```python
from build123d import *

# Parameters (mm, degrees)
SKETCH1_W                 = 130
SKETCH1_H                 = 110
BOSS_EXTRUDE1_DEPTH       = 145
SHELL2_T                  = -5
SHELL2_THICKNESS_2_FACE_W = 100
SHELL2_THICKNESS_2_FACE_H = 120
SHELL2_THICKNESS_2_DEPTH  = 5
SKETCH2_R                 = 23
BOSS_EXTRUDE2_DEPTH       = 12
SKETCH2_3_R               = 25
BOSS_EXTRUDE3_DEPTH       = 13
SKETCH3_R                 = 16
CUT_EXTRUDE1_DEPTH        = 10
SKETCH4_R                 = 17.5
CUT_EXTRUDE4_DEPTH        = 11
SKETCH5_R                 = 5.5
SKETCH5_R_2               = 7
CUT_EXTRUDE5_DEPTH        = 194.261480901
SKETCH7_R                 = 4.25
CUT_EXTRUDE6_DEPTH        = 10
FILLET1_R                 = 3
FILLET2_R                 = 2


with BuildPart() as part:
    # Sketch1 → Boss-Extrude1 (new body)
    with BuildSketch(Plane(origin=(0, 0, 0), x_dir=(0, 1, 0), z_dir=(0, 0, 1))):
        Rectangle(SKETCH1_W, SKETCH1_H)
    extrude(amount=BOSS_EXTRUDE1_DEPTH)

    # Shell2
    shell2_openings = [part.faces().sort_by_distance(p)[0] for p in [
        (0, 0, 145),
    ]]
    offset(amount=SHELL2_T, openings=shell2_openings, kind=Kind.INTERSECTION)

    # Shell2 thickness 2 face (on inner face of the shell) → Shell2 thickness 2 (add)
    with BuildSketch(Plane(origin=(0, 0, 5), x_dir=(-1, 0, 0), z_dir=(0, 0, -1))):
        Rectangle(SHELL2_THICKNESS_2_FACE_W, SHELL2_THICKNESS_2_FACE_H)
    extrude(amount=-SHELL2_THICKNESS_2_DEPTH)

    # Sketch2 → Boss-Extrude2 (add)
    with BuildSketch(Plane.YZ.offset(-50)):
        with Locations((-31, 75)):
            Circle(SKETCH2_R)
    boss_extrude2 = extrude(amount=BOSS_EXTRUDE2_DEPTH)

    # Sketch2_3 → Boss-Extrude3 (add)
    with BuildSketch(Plane.YZ.offset(-50)):
        with Locations(Location((23, 75, 0), (0, 0, 180))):
            Circle(SKETCH2_3_R)
    boss_extrude3 = extrude(amount=BOSS_EXTRUDE3_DEPTH)

    # Sketch3 → Cut-Extrude1 (cut)
    with BuildSketch(Plane.YZ.offset(-38)):
        with Locations((-31, 75)):
            Circle(SKETCH3_R)
    cut_extrude1 = extrude(amount=-CUT_EXTRUDE1_DEPTH, mode=Mode.SUBTRACT)

    # Sketch4 → Cut-Extrude4 (cut)
    with BuildSketch(Plane.YZ.offset(-37)):
        with Locations((23, 75)):
            Circle(SKETCH4_R)
    cut_extrude4 = extrude(amount=-CUT_EXTRUDE4_DEPTH, mode=Mode.SUBTRACT)

    # Mirror1: Boss-Extrude2, Boss-Extrude3, Cut-Extrude1, Cut-Extrude4 across plane
    add(boss_extrude2.mirror(Plane(origin=(0, 0, 0), x_dir=(0, 0, 1), z_dir=(1, 0, 0))))
    add(boss_extrude3.mirror(Plane(origin=(0, 0, 0), x_dir=(0, 0, 1), z_dir=(1, 0, 0))))
    add(cut_extrude1.mirror(Plane(origin=(0, 0, 0), x_dir=(0, 0, 1), z_dir=(1, 0, 0))), mode=Mode.SUBTRACT)
    add(cut_extrude4.mirror(Plane(origin=(0, 0, 0), x_dir=(0, 0, 1), z_dir=(1, 0, 0))), mode=Mode.SUBTRACT)

    # Sketch5 → Cut-Extrude5 (cut, through all)
    with BuildSketch(Plane(origin=(-55, 0, 0), x_dir=(0, -1, 0), z_dir=(-1, 0, 0))):
        with Locations((31, 75)):
            Circle(SKETCH5_R)
        with Locations((-23, 75)):
            Circle(SKETCH5_R_2)
    extrude(amount=-CUT_EXTRUDE5_DEPTH, mode=Mode.SUBTRACT)

    # Sketch7 → Cut-Extrude6 (cut)
    with BuildSketch(Plane(origin=(0, 0, 0), x_dir=(1, 0, 0), z_dir=(0, 0, -1))):
        with Locations(Location((-40, 50, 0), (0, 0, 180))):
            Circle(SKETCH7_R)
        with Locations(Location((40, 50, 0), (0, 0, 180))):
            Circle(SKETCH7_R)
        with Locations(Location((-40, -50, 0), (0, 0, 180))):
            Circle(SKETCH7_R)
        with Locations(Location((40, -50, 0), (0, 0, 180))):
            Circle(SKETCH7_R)
    extrude(amount=-CUT_EXTRUDE6_DEPTH, mode=Mode.SUBTRACT)

    # Fillet1
    fillet1_edges = [part.edges().sort_by_distance(p)[0] for p in [
        (-50, -60, 77.5),
        (50, -60, 77.5),
        (50, 60, 77.5),
        (-50, 60, 77.5),
        (-55, -65, 72.5),
        (-55, 65, 72.5),
        (55, 65, 72.5),
        (55, -65, 72.5),
    ]]
    fillet(fillet1_edges, radius=FILLET1_R)

    # Fillet2
    fillet2_edges = [part.edges().sort_by_distance(p)[0] for p in [
        (-38, -54, 75),
        (-37, 48, 75),
        (38, -54, 75),
        (37, 48, 75),
    ]]
    fillet(fillet2_edges, radius=FILLET2_R)


solid = part.part
```
Design review of the part built by this model. Coordinates are the model's own, in mm. A direction names the side the tool comes from. Coordinates: 2 decimals unless noted, no trailing zeros. Order: outer loops, then holes, each group sorted by start corner. A loop starts at its lowest first (then second) coordinate and runs counter-clockwise, first axis right, second up. Notation, with made-up numbers: (30, 24) -> (40, 24) arc R27 ccw to (40, 44) -> close; hole circle Ø9 at (39.5, -18.5). An arc over 180 degrees is marked (long way). One line per item, written item: value. Start each with the question number.
Q1. Take a section at B-B, the plane y = 50. State the section outline as (x, z) points.
Q2. Insertion check: pin 1 Ø12.5 at (y, z) = (23, 75) entering from -X; pin 2 Ø6 at (x, y) = (-3.5, -24.5) entering from +Z. Each pin has a flat end and moves straight along its axis. Give the tip position at first contact, or say it passes through.
Q3. Take a section at D-D, the plane x = -26. State the section outline as (y, z) points.
Q4. Take a section at C-C, the plane z = 34.5. State the section outline as (x, y) points, then the cut area to 3 significant figures.
Q5. Take a section at A-A, the plane x = 42. State the section outline as (y, z) points.
Q6. Mouldability with a two-part tool opening along Y and no side actions: class faces 1 (the flat face through (1, 65, 71)), 2 (the cylindrical face through (42.93, -33.083, 90.864)), 3 (the flat face through (48, 31, 75)), 4 (the flat face through (55, -1, 71)) as pulls with the +Y half, pulls with the -Y half, needs draft (parallel to the pull), parting line crosses it, or undercut.
Q7. Tool access review of faces 5 (the cylindrical face through (-44.577, 47.976, 73.901)), 6 (the flat face through (37, 31.63, 59.56)), 7 (the cylindrical face through (-36.63, 47.41, 4.93)): name each direction out of +Z, -Z, +X, -X, +Y, -Y from which nothing blocks a thin tool from reaching the whole face with its end or side.
Q8. For probe 1 along Y at (x, z) = (-40, 3); probe 2 along Z at (x, y) = (-44, -31); probe 3 along Y at (x, z) = (-19, 90), list the stretches that pass through material, from the lowest coordinate up.
Values follow:
1. outline: (-55, 0) -> (-44.25, 0) -> (-44.25, 10) -> (-50, 10) -> (-50, 145) -> (-55, 145) -> close; (-35.75, 0) -> (35.75, 0) -> (35.75, 10) -> (-35.75, 10) -> close; (44.25, 0) -> (55, 0) -> (55, 145) -> (50, 145) -> (50, 10) -> (44.25, 10) -> close
2. pin 1: passes through
2. pin 2: stops at z = 10
3. outline: (-65, 0) -> (65, 0) -> (65, 145) -> (60, 145) -> (60, 10) -> (-60, 10) -> (-60, 145) -> (-65, 145) -> close
4. outline: (-55, -62) arc R3 ccw to (-52, -65) -> (52, -65) arc R3 ccw to (55, -62) -> (55, 62) arc R3 ccw to (52, 65) -> (-52, 65) arc R3 ccw to (-55, 62) -> close; hole (-50, -57) arc R3 ccw to (-47, -60) -> (47, -60) arc R3 ccw to (50, -57) -> (50, 57) arc R3 ccw to (47, 60) -> (-47, 60) arc R3 ccw to (-50, 57) -> close
4. area: 2,300 mm2
5. outline: (-65, 0) -> (-53.75, 0) -> (-53.75, 10) -> (-60, 10) -> (-60, 145) -> (-65, 145) -> close; circle Ø46 at (-31, 75); (-46.25, 0) -> (46.25, 0) -> (46.25, 10) -> (-46.25, 10) -> close; circle Ø50 at (23, 75); (53.75, 0) -> (65, 0) -> (65, 145) -> (60, 145) -> (60, 10) -> (53.75, 10) -> close; hole circle Ø32 at (-31, 75); hole circle Ø35 at (23, 75)
6. face 1: pulls with the +Y half
6. face 2: undercut
6. face 3: undercut
6. face 4: needs draft
7. face 5: none
7. face 6: +Z
7. face 7: -Z
8. probe 1: y = -65 to -54.25, -45.75 to 45.75, 54.25 to 65
8. probe 2: z = 0 to 10, 52 to 59, 91 to 98
8. probe 3: y = -65 to -60, 60 to 65
